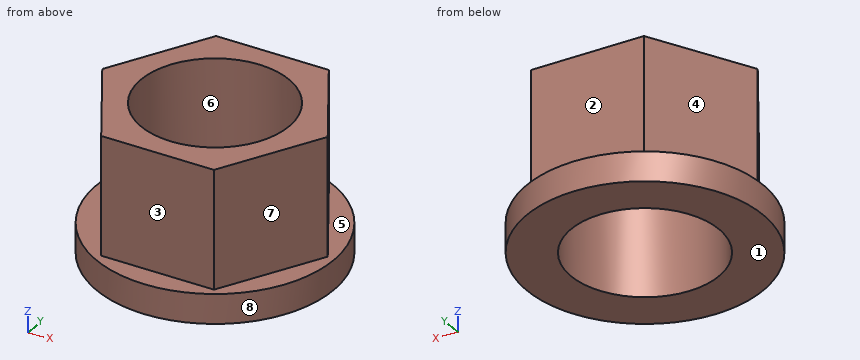
Autodesk Inventor part; units mm, degrees
ref_plane "YZ Plane" through (0, 0, 0) normal (1, 0, 0) x (0, 1, 0)
ref_plane "XZ Plane" through (0, 0, 0) normal (0, 1, 0) x (-1, 0, 0)
ref_plane "XY Plane" through (0, 0, 0) normal (0, 0, 1) x (1, 0, 0)
sketch "草图1" plane through (0, 0, 0) normal (0, 0, 1) x (1, 0, 0)
  circle A0 centre (0, 0) radius 4
  dimension "d0" = 8
extrude "拉伸1" add sketch "草图1" along normal blind 1
sketch "草图2" plane through (0, 0, 1) normal (0, 0, 1) x (1, 0, 0)
  line L0 (1.8764, -3.25) -> (-1.8764, -3.25)
  line L1 (-1.8764, -3.25) -> (-3.7528, 0)
  line L2 (-3.7528, 0) -> (-1.8764, 3.25)
  line L3 (-1.8764, 3.25) -> (1.8764, 3.25)
  line L4 (1.8764, 3.25) -> (3.7528, 0)
  line L5 (3.7528, 0) -> (1.8764, -3.25)
  line L6 (0, 0) -> (0, 3.25)
  dimension "d3" = 6.5
extrude "拉伸2" add sketch "草图2" along normal blind 4
sketch "草图3" plane through (0, 0, 5) normal (0, 0, 1) x (1, 0, 0)
  circle A0 centre (0, 0) radius 2.5
  dimension "d6" = 5
extrude "拉伸3" cut sketch "草图3" against normal through all
thread "螺纹1"
properties part number "分离水箱固定螺帽"
Verification items for the finished model (mm, model axes). Face numbers are marked on the shaded views. A direction names the side the tool comes from. Give positions to 0.01 mm unless a question says otherwise; leave off trailing zeros. Write each loop counter-clockwise with the first axis right and the second up, starting at its lowest first coordinate (ties: lowest second). Pieces come first, ordered by that corner, then holes. Notation, with made-up numbers: (59.25, 40.25) - (107.25, 40.25) arc R18 ccw to (107.25, 73.25) - close; hole circle Ø10 at (51.25, 9). An arc over 180 degrees is marked (long way). Put each result on its own line as item: value.
Q1. Section check D-D on x = -3.5. Record the cut outline in (y, z).
Result:
outline: (-1.94, 0) - (1.94, 0) - (1.94, 1) - (0.44, 1) - (0.44, 5) - (-0.44, 5) - (-0.44, 1) - (-1.94, 1) - close
Q2. Section check C-C on z = 4.2. Record the cut outline in (x, y), and give its area (3 significant figures).
Result:
outline: (-3.75, 0) - (-1.88, -3.25) - (1.88, -3.25) - (3.75, 0) - (1.88, 3.25) - (-1.88, 3.25) - close; hole circle Ø5 at (0, 0)
area: 17.0 mm2
Q3. Section check A-A on x = 0. Record the cut outline in (y, z), and give its area (3 significant figures).
Result:
outline: (-4, 0) - (-2.5, 0) - (-2.5, 5) - (-3.25, 5) - (-3.25, 1) - (-4, 1) - close; (2.5, 0) - (4, 0) - (4, 1) - (3.25, 1) - (3.25, 5) - (2.5, 5) - close
area: 9.00 mm2
Q4. Mould release check, pull along Y, two halves, no side actions. Record for the marked faces 6, 7 and 8: released by +Y, released by -Y, zero draft, split by the parting line, or undercut.
Result:
face 6: undercut
face 7: released by -Y
face 8: split by the parting line
Q5. Set-up check for the marked faces 1, 2, 3, 4 and 5: record each of +Z, -Z, +X, -X, +Y, -Y from which the full face is reachable in a straight line by a thin tool's end or side.
Result:
face 1: -Z, +X, -X, +Y, -Y
face 2: +Z, +X, -X, +Y
face 3: +Z, +X, -X, -Y
face 4: +Z, -X, +Y
face 5: +Z
Q6. Depth check by flat-ended pin: P1, Ø3, axis at x = -0.5, z = 3, coming from the +Y side; P2, Ø3, axis at x = 0.5, y = 0, coming from the -Z side. Enter the tip coordinate at first touch or a pass-through.
Result:
P1: y = 3.25
P2: through
Q7. Section check B-B on y = -1.5. Record the cut outline in (x, z), and give its area (3 significant figures).
Result:
outline: (-3.71, 0) - (-2, 0) - (-2, 5) - (-2.89, 5) - (-2.89, 1) - (-3.71, 1) - close; (2, 0) - (3.71, 0) - (3.71, 1) - (2.89, 1) - (2.89, 5) - (2, 5) - close
area: 10.5 mm2
Q8. Scan lines: probe 1 along Y at (x, z) = (0, 2.35); probe 2 along Z at (x, y) = (-1.25, 3.75); probe 3 along Y at (x, z) = (-2, 3.1). Record each from-to range of solid material in increasing order. Write a range as from..to.
Result:
probe 1: -3.25..-2.5, 2.5..3.25
probe 2: 0..1
probe 3: -3.04..-1.5, 1.5..3.04
